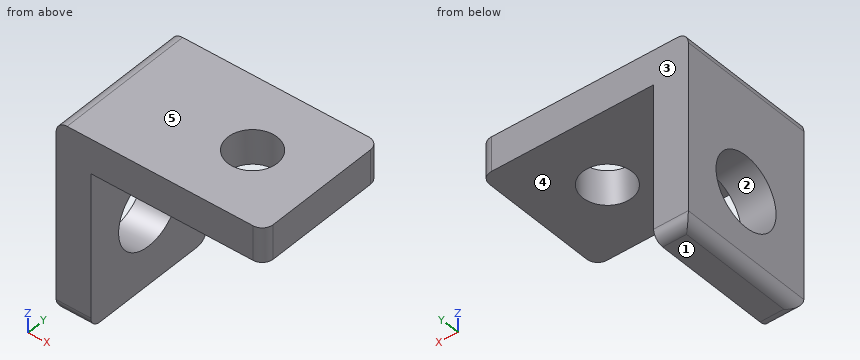
from build123d import *

# Parameters (mm, degrees)
BOSS_EXTRUDE1_DEPTH   = 6.35
CUT_EXTRUDE1_REACH    = 15.388
SKETCH2_R             = 1.651
F_4_40_TAPPED_HOLE2_D = 2.2606
FILLET1_R             = 0.5


with BuildPart() as part:
    # Sketch1 → Boss-Extrude1 (new body)
    with BuildSketch(Plane(origin=(0, 0, 0), x_dir=(1, 0, 0), z_dir=(0, 1, 0))):
        Polygon((0, 8.7122), (0, 0), (9.525, 0), (9.525, 1.5875), (1.5875, 1.5875), (1.5875, 8.7122), align=None)
    extrude(amount=BOSS_EXTRUDE1_DEPTH)

    # Sketch2 → Cut-Extrude1 (cut, up to next)
    with BuildSketch(Plane(origin=(1.5875, 0, 0), x_dir=(0, 0, -1), z_dir=(1, 0, 0)), mode=Mode.PRIVATE) as cut_extrude1_sk1:
        with Locations((5.3, 3.175)):
            Circle(SKETCH2_R)
    cut_extrude1_tool1 = extrude(cut_extrude1_sk1.sketch, amount=-CUT_EXTRUDE1_REACH, mode=Mode.PRIVATE) & part.part
    add(cut_extrude1_tool1.solids().sort_by_distance((1.5875, 3.175, -5.3))[0], mode=Mode.SUBTRACT)

    # #4-40 Tapped Hole2 (through all)
    with Locations(Plane(origin=(6.35, 3.175, -1.5875), x_dir=(-1, 0, 0), z_dir=(0, 0, -1))):
        with Locations((0, 0)):
            Hole(F_4_40_TAPPED_HOLE2_D / 2)

    # Fillet1
    fillet1_edges = [part.edges().sort_by_distance(p)[0] for p in [
        (0, 3.175, 0),
        (0, 3.175, -8.7122),
        (9.525, 6.35, -0.79375),
        (9.525, 0, -0.79375),
        (0.79375, 6.35, -8.7122),
        (0.79375, 0, -8.7122),
    ]]
    fillet(fillet1_edges, radius=FILLET1_R)


solid = part.part
Could you check a few things on this model? Use its own coordinates, in mm. Face numbers are marked on the shaded views. A direction names the side the tool comes from. Give positions to 0.01 mm unless a question says otherwise; leave off trailing zeros. Write each loop counter-clockwise with the first axis right and the second up, starting at its lowest first coordinate (ties: lowest second). Pieces come first, ordered by that corner, then holes. Notation, with made-up numbers: (39, -32.75) - (91, -32.75) arc R22 cw to (91, -13.75) - close; hole circle Ø9 at (-35.5, 31). An arc over 180 degrees is marked (long way). Use CSV: the item, a comma, the result in double quotes. Start each with the question number.
Item 1: I want a section at C-C, the plane y = 3. Please give me the cut outline in (x, z) (1 decimal).
Item 2: If I drill on line 1 along Z through (x, y) = (0.5, 3.25); line 2 along Y through (x, z) = (6.35, -1); line 3 along Z through (x, y) = (4, 5.5), over which ranges is the centre line in solid material (lowest first)?
Item 3: I want a section at D-D, the plane y = 4.5. Please give me the cut outline in (x, z) (1 decimal), then the cut area to 3 significant figures.
Item 4: For the marked faces 4 and 5, which set-ups out of +Z, -Z, +X, -X, +Y, -Y let a thin tool reach every point of the face, with its end or its side?
Item 5: I want a section at A-A, the plane z = -5.3. Please give me the cut outline in (x, y), then the cut area to 3 significant figures.
Item 6: I want a section at B-B, the plane x = 6.35. Please give me the cut outline in (y, z), then the cut area to 3 significant figures.
Item 7: If we mould it in two halves opening along Y, with no side actions, what happens to the marked faces 1, 2 and 3? For each: pulls with the +Y half, pulls with the -Y half, needs draft (parallel to the pull), parting line crosses it, or undercut.
Item 8: I'm going to push flat-ended pins straight in: pin 1 (3 mm diameter, centred on x = 6.35, y = 3.175, fed in from +Z); pin 2 (1 mm diameter, centred on x = 2.5, y = 4, fed in from -Z); pin 3 (3 mm diameter, centred on x = 5, z = -6.5, fed in from +Y); pin 4 (3 mm diameter, centred on y = 0.5, z = -6.5, fed in from +X). Where does each tip first touch, or does it pass through?
Findings:
1,outline,"(0, -8.2) arc R0.5 ccw to (0.5, -8.7) - (1.6, -8.7) - (1.6, -6.9) - (0, -6.9) - close; (0, -3.7) - (1.6, -3.7) - (1.6, -1.6) - (5.2, -1.6) - (5.2, 0) - (0.5, 0) arc R0.5 ccw to (0, -0.5) - close; (7.5, -1.6) - (9.5, -1.6) - (9.5, 0) - (7.5, 0) - close"
2,line 1,"z = -8.71 to -6.95, -3.65 to 0"
2,line 2,"y = 0 to 2.04, 4.31 to 6.35"
2,line 3,"z = -1.59 to 0"
3,outline,"(0, -8.2) arc R0.5 ccw to (0.5, -8.7) - (1.6, -8.7) - (1.6, -6.3) - (0, -6.3) - close; (0, -4.3) - (1.6, -4.3) - (1.6, -1.6) - (9.5, -1.6) - (9.5, 0) - (0.5, 0) arc R0.5 ccw to (0, -0.5) - close"
3,area,"23.2 mm2"
4,face 4,"-Z, +X, +Y, -Y"
4,face 5,"+Z, +X, -X, +Y, -Y"
5,outline,"(0, 0) - (1.59, 0) - (1.59, 1.52) - (0, 1.52) - close; (0, 4.83) - (1.59, 4.83) - (1.59, 6.35) - (0, 6.35) - close"
5,area,"4.84 mm2"
6,outline,"(0, -1.59) - (2.04, -1.59) - (2.04, 0) - (0, 0) - close; (4.31, -1.59) - (6.35, -1.59) - (6.35, 0) - (4.31, 0) - close"
6,area,"6.49 mm2"
7,face 1,"needs draft"
7,face 2,"undercut"
7,face 3,"pulls with the +Y half"
8,pin 1,"stops at z = 0"
8,pin 2,"stops at z = -1.59"
8,pin 3,"passes through"
8,pin 4,"stops at x = 1.59"
